from build123d import *

# Parameters (mm, degrees)
SKETCH1_W           = 13.36
SKETCH1_H           = 7.23
BOSS_EXTRUDE1_DEPTH = 13.325
SKETCH2_W           = 5.5
SKETCH2_H           = 5.5
CUT_EXTRUDE1_DEPTH  = 10
CUT_EXTRUDE2_START  = -11.75
SKETCH3_R           = 2.75
CUT_EXTRUDE2_DEPTH  = 11.75
BOSS_EXTRUDE2_DEPTH = 1.8
BOSS_EXTRUDE3_DEPTH = 1.33
FILLET1_R           = 1


with BuildPart() as part:
    # Sketch1 → Boss-Extrude1 (new, symmetric)
    with BuildSketch(Plane(origin=(0, 0, 0), x_dir=(1, 0, 0), z_dir=(0, 1, 0))):
        Rectangle(SKETCH1_W, SKETCH1_H)
    extrude(amount=BOSS_EXTRUDE1_DEPTH, both=True)

    # Sketch2 → Cut-Extrude1 (cut)
    with BuildSketch(Plane(origin=(0, 13.325, 0), x_dir=(1, 0, 0), z_dir=(0, 1, 0))):
        with BuildLine():
            Line((-5.815, 2.75), (-0.315, 2.75))
            Line((-0.315, 2.75), (-0.315, 0))
            ThreePointArc((-0.315, 0), (-3.065, -2.75), (-5.815, 0))
            Line((-5.815, 0), (-5.815, 2.75))
        make_face()
        with Locations((3.065, 0)):
            Rectangle(SKETCH2_W, SKETCH2_H)
    extrude(amount=-CUT_EXTRUDE1_DEPTH, mode=Mode.SUBTRACT)

    # Sketch3 → Cut-Extrude2 (cut)
    with BuildSketch(Plane.XZ.offset(13.325).offset(CUT_EXTRUDE2_START)):
        with Locations(Location((-3.065, 0, 0), (0, 0, 270))):
            Circle(SKETCH3_R)
        with Locations(Location((3.065, 0, 0), (0, 0, 270))):
            Circle(SKETCH3_R)
    extrude(amount=CUT_EXTRUDE2_DEPTH, mode=Mode.SUBTRACT)

    # Sketch4 → Boss-Extrude2 (add, symmetric)
    with BuildSketch(Plane(origin=(0, 0, 0), x_dir=(0, 0, -1), z_dir=(1, 0, 0))):
        Polygon((3.615, 13.325), (5.145, 10.975), (3.615, 10.975), align=None)
    extrude(amount=BOSS_EXTRUDE2_DEPTH, both=True)

    # Sketch5 → Boss-Extrude3 (add)
    with BuildSketch(Plane(origin=(0, -0.215, 0), x_dir=(1, 0, 0), z_dir=(0, 1, 0))):
        with BuildLine():
            Line((-5.37, 4.925), (-4.56, 4.925))
            ThreePointArc((-4.56, 4.925), (-3.633690117, 4.541309883), (-3.25, 3.615))
            Line((-3.25, 3.615), (-6.68, 3.615))
            ThreePointArc((-6.68, 3.615), (-6.296309883, 4.541309883), (-5.37, 4.925))
        make_face()
        with BuildLine():
            Line((4.56, 4.925), (5.37, 4.925))
            ThreePointArc((5.37, 4.925), (6.296309883, 4.541309883), (6.68, 3.615))
            Line((6.68, 3.615), (3.25, 3.615))
            ThreePointArc((3.25, 3.615), (3.633690117, 4.541309883), (4.56, 4.925))
        make_face()
        with BuildLine():
            Line((-2.36, -4.925), (2.36, -4.925))
            ThreePointArc((2.36, -4.925), (3.286309883, -4.541309883), (3.67, -3.615))
            Line((3.67, -3.615), (-3.67, -3.615))
            ThreePointArc((-3.67, -3.615), (-3.286309883, -4.541309883), (-2.36, -4.925))
        make_face()
    extrude(amount=BOSS_EXTRUDE3_DEPTH)

    # Fillet1
    fillet1_edges = [part.edges().sort_by_distance(p)[0] for p in [
        (-6.68, -6.77, -3.615),
        (6.68, -6.77, -3.615),
        (6.68, 0, 3.615),
        (-6.68, 0, 3.615),
        (-6.68, 7.22, -3.615),
        (6.68, 7.22, -3.615),
    ]]
    fillet(fillet1_edges, radius=FILLET1_R)


solid = part.part
Model file for the job. Use its own axes, mm. A direction names the side the tool comes from. Give positions to 0.01 mm unless a question says otherwise; leave off trailing zeros. Order: outer loops, then holes, each group sorted by start corner. A loop starts at its lowest first (then second) coordinate and runs counter-clockwise, first axis right, second up. Notation, with made-up numbers: (69.25, 12.25) - (89.25, 12.25) arc R23 cw to (89.25, 40.25) - close; hole circle Ø11 at (15, 45.25). An arc over 180 degrees is marked (long way). Return JSON: item names as keys, results as strings.
1) Pull direction Z, two halves, no side cores. Call faces 4 (the cylindrical face through (-3.3, 0.44, 4.53)), 5 (the flat face through (-5.815, 8, -1)), 6 (the flat face through (5, 1.115, -4)): pulls with the +Z half, pulls with the -Z half, needs draft (parallel to the pull), parting line crosses it, or undercut.
Geometry says:
{"face 4": "pulls with the +Z half", "face 5": "undercut", "face 6": "needs draft"}
2) Cut at C-C, the plane x = 1.5. Give the cut face in (y, z) (3 decimals), plus the area to 3 significant figures.
Geometry says:
{"outline": "(-13.325, -3.615) - (10.975, -3.615) - (10.975, -5.145) - (13.325, -3.615) - (13.325, -2.75) - (3.325, -2.75) - (3.325, 2.75) - (13.325, 2.75) - (13.325, 3.615) - (1.115, 3.615) - (1.115, 4.925) - (-0.215, 4.925) - (-0.215, 3.615) - (-13.325, 3.615) - (-13.325, 2.261) - (-1.575, 2.261) - (-1.575, -2.261) - (-13.325, -2.261) - close", "area": "88.1 mm²"}
3) Cut at B-B, the plane z = -3.25. Give the cut face in (x, y) (3 decimals).
Geometry says:
{"outline": "(-6.68, -0.215) - (-6.453, -0.215) - (-6.453, -13.325) - (6.453, -13.325) - (6.453, -0.215) - (6.68, -0.215) - (6.68, 1.115) - (6.453, 1.115) - (6.453, 13.325) - (-6.453, 13.325) - (-6.453, 1.115) - (-6.68, 1.115) - close"}
4) Probe line 1 (X direction, y = -7.25, z = 0) (3 decimals); line 2 (X direction, y = -10.5, z = -2.5); line 3 (Z direction, x = 3, y = -2.5) (3 decimals). List the from-to ranges inside material, lowest first. Write a range as from..to.
Geometry says:
{"line 1": "-6.68..-5.815, -0.315..0.315, 5.815..6.68", "line 2": "-6.68..-4.21, -1.92..1.92, 4.21..6.68", "line 3": "-3.615..-2.749, 2.749..3.615"}
5) 3-axis set-ups, long thin cutter, end or side, ignore diameter. For faces 1 (the flat face through (5, 0, -4.925)), 2 (the flat face through (0, 1.115, 4)), 3 (the flat face through (-0.315, 8, -1)): which of +Z, -Z, +X, -X, +Y, -Y reach the whole face in a straight line?
Geometry says:
{"face 1": "-Z, +X, -X, +Y, -Y", "face 2": "+Z, +X, -X, +Y", "face 3": "+Y"}
6) Flat gauge pins, fed straight in: P1, Ø3.5, axis at x = 2, y = 3, coming from the +Z side (3 decimals); P2, Ø6, axis at x = 4.5, y = 1, coming from the -Z side (3 decimals); P3, Ø1.6, axis at x = -2, z = 0, coming from the +Y side (3 decimals). Where does each tip first touch, or does it go through?
Geometry says:
{"P1": "z = 3.615", "P2": "z = -4.925", "P3": "y = 3.325"}
7) Cut at A-A, the plane y = 9. Give the cut face in (x, z) (3 decimals), plus the area to 3 significant figures.
Geometry says:
{"outline": "(-6.68, -2.615) arc R1 ccw to (-5.68, -3.615) - (5.68, -3.615) arc R1 ccw to (6.68, -2.615) - (6.68, 2.615) arc R1 ccw to (5.68, 3.615) - (-5.68, 3.615) arc R1 ccw to (-6.68, 2.615) - close; hole (-5.815, -2.75) - (-0.315, -2.75) - (-0.315, 0) arc R2.75 ccw to (-5.815, 0) - close; hole (0.315, -2.75) - (5.815, -2.75) - (5.815, 2.75) - (0.315, 2.75) - close", "area": "38.5 mm²"}
8) Cut at D-D, the plane z = 2. Give the cut face in (x, y) (3 decimals), plus the area to 3 significant figures.
Geometry says:
{"outline": "(-6.68, -13.325) - (-4.952, -13.325) - (-4.952, -1.575) - (-1.178, -1.575) - (-1.178, -13.325) - (1.178, -13.325) - (1.178, -1.575) - (4.952, -1.575) - (4.952, -13.325) - (6.68, -13.325) - (6.68, 13.325) - (5.815, 13.325) - (5.815, 3.325) - (0.315, 3.325) - (0.315, 13.325) - (-1.178, 13.325) - (-1.178, 3.325) - (-4.952, 3.325) - (-4.952, 13.325) - (-6.68, 13.325) - close", "area": "175 mm²"}
